Autodesk Inventor part; units mm, degrees
ref_plane "YZ Plane" through (0, 0, 0) normal (1, 0, 0) x (0, 1, 0)
ref_plane "XZ Plane" through (0, 0, 0) normal (0, 1, 0) x (-1, 0, 0)
ref_plane "XY Plane" through (0, 0, 0) normal (0, 0, 1) x (1, 0, 0)
sketch "Sketch1" plane through (0, 0, 0) normal (0, 1, 0) x (-1, 0, 0)
  line L0 (0, 0) -> (296.8625, 0)
  line L1 (296.8625, 0) -> (296.8625, -525.4625)
  line L2 (296.8625, -525.4625) -> (0, -525.4625)
  line L3 (0, -525.4625) -> (0, 0)
  line L4 (308.7687, 9.525) -> (-11.9063, 9.525)
  line L5 (-11.9063, 9.525) -> (-11.9062, -534.9875)
  line L6 (-11.9062, -534.9875) -> (308.7688, -534.9875)
  line L7 (308.7688, -534.9875) -> (308.7687, 9.525)
  dimension "d0" = 296.8625
  dimension "d1" = 525.4625
  dimension "d4" = 11.9062
  dimension "d5" = 11.9062
  dimension "d6" = 9.525
  dimension "d7" = 9.525
extrude "Extrusion1" add sketch "Sketch1" along normal blind 9.7282 contours L0 L1 L2 L3 | L7 L6 L5 L4
sketch "Sketch2" plane through (0, 9.7282, 0) normal (0, 1, 0) x (1, 0, 0)
  line L0 (-296.8562, 0) -> (-0.0063, 0)
  line L1 (-0.0063, 0) -> (-0.0064, 525.4625)
  line L2 (-0.0064, 525.4625) -> (-296.8562, 525.4625)
  line L3 (-296.8562, 525.4625) -> (-296.8562, 0)
  line L4 (-308.7688, 534.9875) -> (-308.7687, -9.525)
  line L5 (-308.7687, -9.525) -> (11.9063, -9.525)
  line L6 (11.9062, 534.9875) -> (-308.7688, 534.9875)
  line L7 (11.9063, -9.525) -> (11.9062, 534.9875)
  point P0 (0, 0)
  dimension "d10" = 11.9126
  dimension "d11" = 9.525
  dimension "d12" = 9.525
  dimension "d13" = 11.9126
extrude "Extrusion2" cut sketch "Sketch2" against normal blind 1.5875 contours L3 L2 L1 L0
properties part number "LCD Screen"
CAD build for the part. Positions are in the model's coordinates, mm. Give positions to 0.01 mm unless a question says otherwise; leave off trailing zeros. Loops run counter-clockwise (first coordinate to the right, second up) from the corner with the lowest first, then second, coordinate; pieces in that order, holes last. Notation, with made-up numbers: (82.5, 61) - (111.5, 61) arc R19 ccw to (111.5, 80) - close; hole circle Ø6 at (31, 82). An arc over 180 degrees is marked (long way). Put each result on its own line as item: value.
Q1. Mould opens along X. For faces 1 (the face through (-151, 8.141, -266)), 2 (the face through (7, 9.728, -181)), 3 (the face through (-308.769, 5, -267)) say: pulls with the +X half, pulls with the -X half, needs draft (parallel to the pull), parting line crosses it, or undercut.
Filled in:
face 1: undercut
face 2: needs draft
face 3: pulls with the -X half
Q2. Slice it at A-A (x = -23). Give the cut face in (y, z) (1 decimal), plus the area to 3 significant figures.
Filled in:
outline: (0, -535) - (9.7, -535) - (9.7, -525.5) - (8.1, -525.5) - (8.1, 0) - (9.7, 0) - (9.7, 9.5) - (0, 9.5) - close
area: 4,460 mm²
Q3. Slice it at B-B (z = -367.5). Give the cut face in (x, y).
Filled in:
outline: (-308.77, 0) - (11.91, 0) - (11.91, 9.73) - (-0.01, 9.73) - (-0.01, 8.14) - (-296.86, 8.14) - (-296.86, 9.73) - (-308.77, 9.73) - close
Q4. Probe line 1 along X through (y, z) = (9, -352); line 2 along Z through (x, y) = (-4.5, 8.5) (1 decimal); line 3 along Y through (x, z) = (-108, -361). List the from-to ranges inside material, lowest first.
Filled in:
line 1: x = -308.77 to -296.86, -0.01 to 11.91
line 2: z = -535 to -525.5, 0 to 9.5
line 3: y = 0 to 8.14
Q5. Flat gauge pin, fed straight in: pin 1 (1 mm diameter, centred on x = -68.5, z = -126, fed in from +Y). Where does the tip first touch, or does it go through?
Filled in:
pin 1: stops at y = 8.14
